Could you check a few things on this model? Use its own coordinates, in mm. Give positions to 0.01 mm unless a question says otherwise; leave off trailing zeros. Order: outer loops, then holes, each group sorted by start corner. A loop starts at its lowest first (then second) coordinate and runs counter-clockwise, first axis right, second up. Notation, with made-up numbers: M -21,9.5 L 29,9.5 A31 ccw 29,35.5 Z; hole C -27.5,1 d8. An arc over 180 degrees is marked long. Return JSON: item names as keys, results as strings. Group by question number.
```python
from build123d import *

# Parameters (mm, degrees)
F1_DEPTH = 10
F2_R     = 1


with BuildPart() as f1:
    # F0 (on Front) → F1 (new body, symmetric)
    with BuildSketch(Plane.XZ):
        Polygon((0, 20), (0, 0), (100, 0), align=None)
    extrude(amount=F1_DEPTH, both=True)

    # F2
    f2_edges = [f1.edges().sort_by_distance(p)[0] for p in [
        (50, -10, 10),
        (50, 10, 10),
        (0, 0, 20),
        (0, -10, 10),
        (0, 10, 10),
    ]]
    fillet(f2_edges, radius=F2_R)


solid = f1.part
```
1. For pin 1 (12 mm diameter, centred on x = 65.5, y = 3.5, fed in from +Z); pin 2 (5 mm diameter, centred on x = 21.5, y = 7, fed in from +Z), each with a flat end and sliding along its axis, tell me the tip position at first contact or that it passes through.
2. Imagine slicing it at A-A, the plane y = -0.25. Please give me the cut outline in (x, z), plus the area to 4 significant figures.
3. I need wall thicknesses on L1, parallel to Z at x = 66, y = 1.25; L2, parallel to Z at x = 95.5, y = 3.25. Which ranges of each line are inside material? Lowest first, please. Write a range as from..to.
Values:
{
 "1": {"pin 1": "stops at z = 8.1", "pin 2": "stops at z = 16.2"},
 "2": {"outline": "M 0,0 L 100,0 L 1.2,19.76 A1 ccw 0,18.78 Z", "area": "1,000 mm²"},
 "3": {"L1": "z = 0..6.8", "L2": "z = 0..0.9"}
}
